Can you work these out from the model? Positions are in its coordinate system, mm. A direction names the side the tool comes from. Give positions to 0.01 mm unless a question says otherwise; leave off trailing zeros. Loops run counter-clockwise (first coordinate to the right, second up) from the corner with the lowest first, then second, coordinate; pieces in that order, holes last. Notation, with made-up numbers: (33.25, 28) -> (56.25, 28) arc R12 ccw to (56.25, 42) -> close; hole circle Ø2 at (54.25, 25). An arc over 180 degrees is marked (long way). Return JSON: item names as keys, results as strings. Group by question number.
Q1. I need wall thicknesses on line 1 along X through (y, z) = (-2.5, -3.5); line 2 along X through (y, z) = (-1.5, -2.5); line 3 along Z through (x, y) = (-21.5, 1.75). Which ranges of each line are inside material? Lowest first, please. Write a range as [from, to].
Q2. Suppose I cut it at C-C, the plane x = -15.25. Please give me the cut outline in (y, z).
Q3. Suppose I cut it at D-D, the plane z = -0.5. Please give me the cut outline in (x, y), and give its area (3 significant figures).
Q4. Which directions (+Z, -Z, +X, -X, +Y, -Y) give clear straight access to the entire face, cutting with the end or side of a thin tool? Please do faces 1 (the flat face through (-22, -3, 0)), 2 (the flat face through (-22, 0, 3)), 3 (the flat face through (-7, 0, 0)), 4 (the flat face through (-22, 0, -3)).
Q5. Will these pins go through, and if not, where does the flat tip stop? pin 1 (3 mm diameter, centred on y = -4.5, z = -3.5, fed in from -X); pin 2 (1 mm diameter, centred on x = -11, y = -3.5, fed in from -Z); pin 3 (3 mm diameter, centred on x = -21, y = 0, fed in from -Z).
Q6. Suppose I cut it at B-B, the plane y = 0. Please give me the cut outline in (x, z), and give its area (3 significant figures).
Q7. Suppose I cut it at A-A, the plane x = -6. Please give me the cut outline in (y, z).
```python
from build123d import *

# Parameters (mm, degrees)
STOCK_STICK_1_START       = -19
STOCK_STICK_1_OUTLINE_R   = 6
STOCK_STICK_1_DEPTH       = 19
STOCK_STICK_1_START_2     = -25
STOCK_STICK_1_2_OUTLINE_W = 6
STOCK_STICK_1_2_OUTLINE_H = 6
STOCK_STICK_1_2_DEPTH     = 6
SKETCH1_W                 = 5.1
SKETCH1_H                 = 5.1
CUT_EXTRUDE1_DEPTH        = 7


# Read off the part's stored shape, not the designer's step: Stock-Stick-1
with BuildPart() as part:
    # Stock-Stick-1 outline → Stock-Stick-1 (new body)
    with BuildSketch(Plane.YZ.offset(STOCK_STICK_1_START)):
        Circle(STOCK_STICK_1_OUTLINE_R)
    extrude(amount=STOCK_STICK_1_DEPTH)

    # Stock-Stick-1 2 outline → Stock-Stick-1 2 (add)
    with BuildSketch(Plane.YZ.offset(STOCK_STICK_1_START_2)):
        Rectangle(STOCK_STICK_1_2_OUTLINE_W, STOCK_STICK_1_2_OUTLINE_H)
    extrude(amount=STOCK_STICK_1_2_DEPTH)

    # Sketch1 → Cut-Extrude1 (cut)
    with BuildSketch(Plane(origin=(0, 0, 0), x_dir=(0, 0, -1), z_dir=(1, 0, 0))):
        Rectangle(SKETCH1_W, SKETCH1_H)
    extrude(amount=-CUT_EXTRUDE1_DEPTH, mode=Mode.SUBTRACT)


solid = part.part
```
Ans:
{
 "1": {"line 1": "x = [-19, 0]", "line 2": "x = [-25, -7]", "line 3": "z = [-3, 3]"},
 "2": {"outline": "circle Ø12 at (0, 0)"},
 "3": {"outline": "(-25, -3) -> (-19, -3) -> (-19, -5.98) -> (0, -5.98) -> (0, -2.55) -> (-7, -2.55) -> (-7, 2.55) -> (0, 2.55) -> (0, 5.98) -> (-19, 5.98) -> (-19, 3) -> (-25, 3) -> close", "area": "228 mm^2"},
 "4": {"face 1": "+Z, -Z, -X, -Y", "face 2": "+Z, -X, +Y, -Y", "face 3": "+X", "face 4": "-Z, -X, +Y, -Y"},
 "5": {"pin 1": "stops at x = -19", "pin 2": "stops at z = -5.2", "pin 3": "stops at z = -3"},
 "6": {"outline": "(-25, -3) -> (-19, -3) -> (-19, -6) -> (0, -6) -> (0, -2.55) -> (-7, -2.55) -> (-7, 2.55) -> (0, 2.55) -> (0, 6) -> (-19, 6) -> (-19, 3) -> (-25, 3) -> close", "area": "228 mm^2"},
 "7": {"outline": "circle Ø12 at (0, 0); hole (-2.55, -2.55) -> (2.55, -2.55) -> (2.55, 2.55) -> (-2.55, 2.55) -> close"}
}
